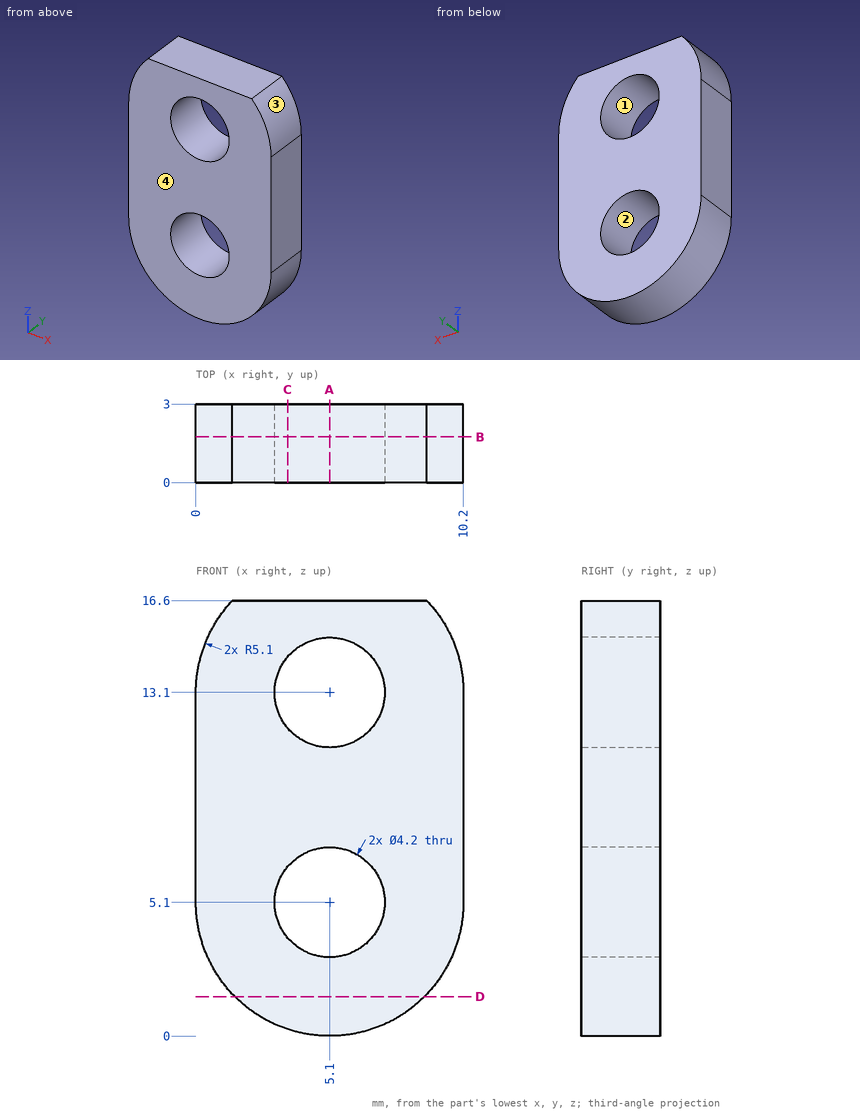
Design review of the part shown in the three views and the two pictorial views. Dimensions are in mm from the part's minimum x, y and z. Coordinates: 2 decimals unless noted, no trailing zeros. Order: outer loops, then holes, each group sorted by start corner. A loop starts at its lowest first (then second) coordinate and runs counter-clockwise, first axis right, second up. Notation, with made-up numbers: (-37, 42.25) - (-7, 42.25) arc R16 ccw to (-7, 59.25) - close; hole circle Ø1 at (67.25, -39.5). An arc over 180 degrees is marked (long way). One line per question, with ' | ' between items.
Q1. Consider section C-C, the plane x = 3.5. Give the boundary of the cut face in (y, z), then the cut area to 3 significant figures.
Answer key:
outline: (0, 0.26) - (3, 0.26) - (3, 3.74) - (0, 3.74) - close; (0, 6.46) - (3, 6.46) - (3, 11.74) - (0, 11.74) - close; (0, 14.46) - (3, 14.46) - (3, 16.6) - (0, 16.6) - close | area: 32.7 mm2
Q2. Clearance check with flat-ended pins moving along their axes: pin 1 Ø1.5 at (x, z) = (5.5, 4.5) entering from -Y; pin 2 Ø1.5 at (y, z) = (2.5, 2) entering from -X. State where each tip first meets the part, or that it passes through.
Answer key:
pin 1: passes through | pin 2: stops at x = 0.57
Q3. Consider section D-D, the plane z = 1.5. Give the boundary of the cut face in (x, y).
Answer key:
outline: (1.49, 0) - (8.71, 0) - (8.71, 3) - (1.49, 3) - close
Q4. Consider section B-B, the plane y = 1.75. Give the boundary of the cut face in (x, z), then the cut area to 3 significant figures.
Answer key:
outline: (0, 5.1) arc R5.1 ccw to (10.2, 5.1) - (10.2, 13.1) arc R5.1 ccw to (8.81, 16.6) - (1.39, 16.6) arc R5.1 ccw to (0, 13.1) - close; hole circle Ø4.2 at (5.1, 5.1); hole circle Ø4.2 at (5.1, 13.1) | area: 127 mm2
Q5. To check wall thickness, follow line 1 along Z through (x, y) = (5.1, 1.3); line 2 along Z through (x, y) = (7, 2.95); line 3 along X through (y, z) = (2.6, 4.25). State the ranges of each line that lie inside material, in increasing order.
Answer key:
line 1: z = 0 to 3, 7.2 to 11, 15.2 to 16.6 | line 2: z = 0.37 to 4.21, 5.99 to 12.21, 13.99 to 16.6 | line 3: x = 0.07 to 3.18, 7.02 to 10.13
Q6. The part is to be moulded in two halves that separate along Z. For the marked faces 1, 2, 3 and 4, say which applies: +Z half, -Z half, draft (parallel to the pull), parting line (faces both ways), or undercut.
Answer key:
face 1: undercut | face 2: undercut | face 3: +Z half | face 4: draft
Q7. Consider section A-A, the plane x = 5.1. Give the boundary of the cut face in (y, z), then the cut area to 3 significant figures.
Answer key:
outline: (0, 0) - (3, 0) - (3, 3) - (0, 3) - close; (0, 7.2) - (3, 7.2) - (3, 11) - (0, 11) - close; (0, 15.2) - (3, 15.2) - (3, 16.6) - (0, 16.6) - close | area: 24.6 mm2
